For this review, take the finished solid that the model builds, in its own axes (mm). A direction names the side the tool comes from. Give positions to 0.01 mm unless a question says otherwise; leave off trailing zeros. Write each loop counter-clockwise with the first axis right and the second up, starting at its lowest first coordinate (ties: lowest second). Pieces come first, ordered by that corner, then holes.
Q1. We need section B-B (z = 0). Write out the cut boundary in (x, y).
Q2. We need section A-A (y = 0). Write out the cut boundary in (x, z), then the cut area to 3 significant figures.
Q3. We need section C-C (x = 5.5). Write out the cut boundary in (y, z), then the cut area to 3 significant figures.
Q4. Mouldability with a two-part tool opening along Y and no side actions: class faces 1 (the flat face through (3.4, -4, 2)), 2 (the flat face through (18.4, 0, 0)), 3 (the cylindrical face through (0.71, 3.233, 1.341)) as released by +Y, released by -Y, zero draft, split by the parting line, or undercut.
Q5. For line 1 (X direction, y = -0.25, z = 2.75); line 2 (X direction, y = 0.75, z = 3.75); line 3 (Z direction, x = 16.75, y = -0.25), list the stretches that pass through material, from the lowest coordinate up.
Q6. We need section D-D (x = 14). Write out the cut boundary in (y, z).
Q7. Insertion check: P1, Ø5, axis at y = 1.5, z = 0.5, coming from the +X side; P2, Ø2, axis at x = 10.5, y = -0.5, coming from the -Z side; P3, Ø0.9, axis at x = 20.5, z = 0, coming from the +Y side; P4, Ø1, axis at y = -1.5, z = 2.5, coming from the +X side. Each pin has a flat end and moves straight along its axis. Give the tip position at first contact, or say it passes through.
Q8. Machinability: for faces 4 (the flat face through (0, 0, 0)), 5 (the flat face through (20, -2.575, 0)), 6 (the flat face through (20, 2.225, 0)), 7 (the cylindrical face through (7.963, -0.867, 3.905)), 8 (the flat face through (20, 1.925, 0)), which of the approach directions +Z, -Z, +X, -X, +Y, -Y give a long, thin tool a straight path to every point of the face, cutting with its end or side? Answer none if there is none.
```python
from build123d import *

# Parameters (mm, degrees)
CHAMFER_1_SIZE  = 1
SKETCH_2_W      = 1.8
SKETCH_2_H      = 0.3
EXTRUDE_1_DEPTH = 3.5
CHAMFER_2_SIZE  = 0.5


with BuildPart() as part:
    # 草图1 → 旋转1 (revolve)
    with BuildSketch(Plane.XY):
        Polygon((0, 0), (0, 3.5), (1.4, 3.5), (1.4, 5.25), (3.4, 5.25), (3.4, 4), (12.4, 4), (12.4, 3.5), (18.4, 3.5), (18.4, 0), align=None)
    revolve(axis=Axis((18.4, 0, 0), (-1, 0, 0)))

    # 倒角1
    chamfer_1_edges = [part.edges().sort_by_distance(p)[0] for p in [
        (1.4, -5.25, 0),
    ]]
    chamfer(chamfer_1_edges, length=CHAMFER_1_SIZE)

    # 草图2 → 凸台-拉伸1 (add)
    with BuildSketch(Plane(origin=(18.4, 0, 0), x_dir=(0, 0, -1), z_dir=(1, 0, 0))):
        with Locations((0, 2.075060306)):
            Rectangle(SKETCH_2_W, SKETCH_2_H)
        with Locations((0, -2.424939694)):
            Rectangle(SKETCH_2_W, SKETCH_2_H)
    extrude(amount=EXTRUDE_1_DEPTH)

    # 倒角2
    chamfer_2_edges = [part.edges().sort_by_distance(p)[0] for p in [
        (21.9, 2.075060306, 0.9),
        (21.9, 2.075060306, -0.9),
        (21.9, -2.424939694, 0.9),
        (21.9, -2.424939694, -0.9),
    ]]
    chamfer(chamfer_2_edges, length=CHAMFER_2_SIZE)


solid = part.part
```
Computed:
1. outline: (0, -3.5) - (1.4, -3.5) - (1.4, -4.25) - (2.4, -5.25) - (3.4, -5.25) - (3.4, -4) - (12.4, -4) - (12.4, -3.5) - (18.4, -3.5) - (18.4, -2.57) - (21.9, -2.57) - (21.9, -2.27) - (18.4, -2.27) - (18.4, 1.93) - (21.9, 1.93) - (21.9, 2.23) - (18.4, 2.23) - (18.4, 3.5) - (12.4, 3.5) - (12.4, 4) - (3.4, 4) - (3.4, 5.25) - (2.4, 5.25) - (1.4, 4.25) - (1.4, 3.5) - (0, 3.5) - close
2. outline: (0, -3.5) - (1.4, -3.5) - (1.4, -4.25) - (2.4, -5.25) - (3.4, -5.25) - (3.4, -4) - (12.4, -4) - (12.4, -3.5) - (18.4, -3.5) - (18.4, 3.5) - (12.4, 3.5) - (12.4, 4) - (3.4, 4) - (3.4, 5.25) - (2.4, 5.25) - (1.4, 4.25) - (1.4, 3.5) - (0, 3.5) - close
2. area: 144 mm2
3. outline: circle Ø8 at (0, 0)
3. area: 50.3 mm2
4. face 1: zero draft
4. face 2: undercut
4. face 3: split by the parting line
5. line 1: x = 0 to 18.4
5. line 2: x = 1.4 to 12.4
5. line 3: z = -3.49 to 3.49
6. outline: circle Ø7 at (0, 0)
7. P1: stops at x = 21.9
7. P2: stops at z = -4
7. P3: stops at y = 2.23
7. P4: stops at x = 18.4
8. face 4: +Z, -Z, -X, +Y, -Y
8. face 5: +Z, -Z, +X, -Y
8. face 6: +Z, -Z, +X, +Y
8. face 7: +X
8. face 8: +Z, -Z, +X
